from build123d import *

# Parameters (mm, degrees)
SKETCH1_W               = 25.4
SKETCH1_H               = 25.4
SKETCH1_W_2             = 21.4
SKETCH1_H_2             = 21.4
BOSS_EXTRUDE1_DEPTH     = 300
CUT_EXTRUDE1_DEPTH      = 302.341085815
CUT_EXTRUDE1_DEPTH_BACK = 302.341085815
SKETCH2_R               = 2


with BuildPart() as part:
    # Sketch1 → Boss-Extrude1 (new body)
    with BuildSketch(Plane(origin=(0, 0, 0), x_dir=(1, 0, 0), z_dir=(0, 1, 0))):
        Rectangle(SKETCH1_W, SKETCH1_H)
        Rectangle(SKETCH1_W_2, SKETCH1_H_2, mode=Mode.SUBTRACT)
    extrude(amount=BOSS_EXTRUDE1_DEPTH)

    # Sketch2 → Cut-Extrude1 (cut, two sides: drawn at the far end of the back side and taken through both)
    with BuildSketch(Plane.XY.offset(12.7).offset(-CUT_EXTRUDE1_DEPTH_BACK)):
        with Locations((-6, 12.7)):
            Circle(SKETCH2_R)
        with Locations((6, 12.7)):
            Circle(SKETCH2_R)
        with Locations((6, 287.3)):
            Circle(SKETCH2_R)
        with Locations((-6, 287.3)):
            Circle(SKETCH2_R)
    extrude(amount=CUT_EXTRUDE1_DEPTH + CUT_EXTRUDE1_DEPTH_BACK, mode=Mode.SUBTRACT)


solid = part.part
For this review, take the finished solid that the model builds, in its own axes (mm). A direction names the side the tool comes from. Round coordinates to 2 decimals unless told otherwise and drop trailing zeros. Loops run counter-clockwise (first coordinate to the right, second up) from the corner with the lowest first, then second, coordinate; pieces in that order, holes last. Notation, with made-up numbers: (-14, 15) - (20, 15) arc R9 cw to (20, 20) - close; hole circle Ø6 at (55.5, 49). An arc over 180 degrees is marked (long way). Use one line per item in the form item = value.
1) We need section B-B on z = 5.5. Write out the cut boundary in (x, y), then the cut area to 3 significant figures.
Solutions:
outline = (-12.7, 0) - (-10.7, 0) - (-10.7, 300) - (-12.7, 300) - close; (10.7, 0) - (12.7, 0) - (12.7, 300) - (10.7, 300) - close
area = 1,200 mm2
2) Clearance check with a flat-ended pin moving along its axis: P1, Ø6, axis at x = -2, z = -6, coming from the -Y side. State where the tip first meets the part, or that it passes through.
Solutions:
P1 = through
3) Tool access review of faces 5 (the face through (0, 148, 10.7)), 6 (the face through (11, 0, 0)): name each direction out of +Z, -Z, +X, -X, +Y, -Y from which nothing blocks a thin tool from reaching the whole face with its end or side.
Solutions:
face_5 = +Y, -Y
face_6 = +Z, -Z, +X, -X, -Y
4) We need section C-C on y = 250.5. Write out the cut boundary in (x, z), then the cut area to 3 significant figures.
Solutions:
outline = (-12.7, -12.7) - (12.7, -12.7) - (12.7, 12.7) - (-12.7, 12.7) - close; hole (-10.7, -10.7) - (10.7, -10.7) - (10.7, 10.7) - (-10.7, 10.7) - close
area = 187 mm2
5) Wall thickness on probe 1 along Y at (x, z) = (-6, -11.35); probe 2 along X at (y, z) = (12.7, -11.3); probe 3 along X at (y, z) = (93, 1.5): over which ranges is each line inside the solid? List them lowest first.
Solutions:
probe_1 = 0 to 10.7, 14.7 to 285.3, 289.3 to 300
probe_2 = -12.7 to -8, -4 to 4, 8 to 12.7
probe_3 = -12.7 to -10.7, 10.7 to 12.7
6) We need section A-A on x = -1.25. Write out the cut boundary in (y, z).
Solutions:
outline = (0, -12.7) - (300, -12.7) - (300, -10.7) - (0, -10.7) - close; (0, 10.7) - (300, 10.7) - (300, 12.7) - (0, 12.7) - close
7) Mouldability with a two-part tool opening along Z and no side actions: class faces 1 (the face through (11, 300, 0)), 2 (the face through (0, 148, -12.7)), 3 (the face through (0, 148, 12.7)), 4 (the face through (0, 148, -10.7)) as pulls with the +Z half, pulls with the -Z half, needs draft (parallel to the pull), parting line crosses it, or undercut.
Solutions:
face_1 = needs draft
face_2 = pulls with the -Z half
face_3 = pulls with the +Z half
face_4 = undercut
